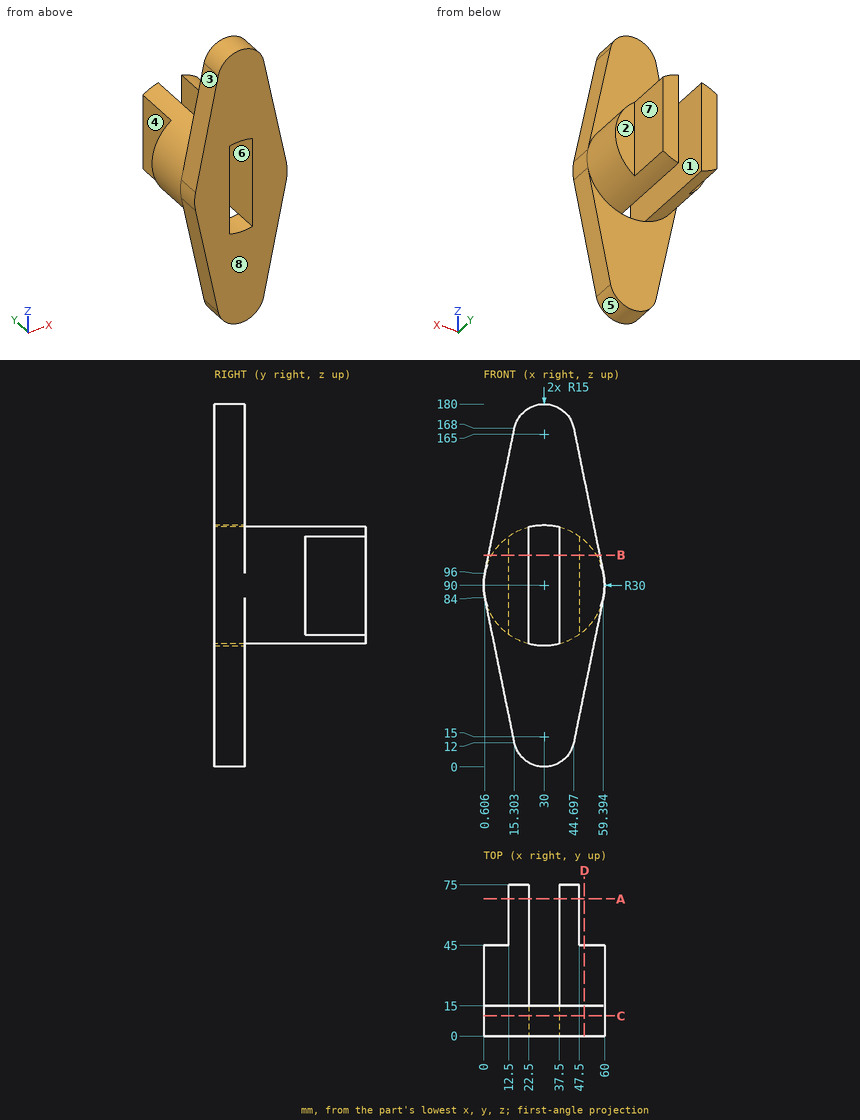
Here's the drawing with two shaded views (mm, measured from the low corner). I have some questions. A direction names the side the tool comes from. Round coordinates to 2 decimals unless told otherwise and drop trailing zeros. Order: outer loops, then holes, each group sorted by start corner. A loop starts at its lowest first (then second) coordinate and runs counter-clockwise, first axis right, second up. Notation, with made-up numbers: M 5.5,6.25 L 15.5,6.25 A18 cw 15.5,14.25 Z; hole C -39,61 d10. An arc over 180 degrees is marked long. Answer in a Markdown table with one row per item.
Item 1: If I drill on L1, parallel to X at y = 51, z = 114; L2, parallel to Y at x = 56.5, z = 86; L3, parallel to Y at x = 8, z = 121, over which ranges is the centre line in solid material (lowest first)? Write a range as from..to.
A:
| item | result |
|---|---|
| L1 | x = 12.5..22.5, 37.5..47.5 |
| L2 | y = 0..45 |
| L3 | y = 0..15 |
Item 2: Imagine slicing it at D-D, the plane x = 50. Write out the boundary of the cut face in (y, z), and give its area (3 significant figures).
A:
| item | result |
|---|---|
| outline | M 0,37.98 L 15,37.98 L 15,67.64 L 45,67.64 L 45,112.36 L 15,112.36 L 15,142.02 L 0,142.02 Z |
| area | 2,900 mm2 |
Item 3: Thinking about a two-plate mould opening in Z: for the marked faces 1, 2 and 3, which applies, +Z half, -Z half, draft (parallel to the pull), parting line (faces both ways), or undercut?
A:
| item | result |
|---|---|
| face 1 | undercut |
| face 2 | draft |
| face 3 | +Z half |
Item 4: Imagine slicing it at B-B, the plane z = 105. Write out the boundary of the cut face in (x, y), and give its area (3 significant figures).
A:
| item | result |
|---|---|
| outline | M 2.44,0 L 22.5,0 L 22.5,75 L 12.5,75 L 12.5,45 L 4.02,45 L 4.02,15 L 2.44,15 Z; M 37.5,0 L 57.56,0 L 57.56,15 L 55.98,15 L 55.98,45 L 47.5,45 L 47.5,75 L 37.5,75 Z |
| area | 2,310 mm2 |
Item 5: Imagine slicing it at C-C, the plane y = 10. Write out the boundary of the cut face in (x, z).
A:
| item | result |
|---|---|
| outline | M 0.61,84 L 15.3,12 A15 ccw 44.7,12 L 59.39,84 A30 ccw 59.39,96 L 44.7,168 A15 ccw 15.3,168 L 0.61,96 A30 ccw Z; hole M 22.5,60.95 A30 ccw 37.5,60.95 L 37.5,119.05 A30 ccw 22.5,119.05 Z |
Item 6: For the marked faces 4, 5, 6, 7 and 8, which set-ups out of +Z, -Z, +X, -X, +Y, -Y let a thin tool reach every point of the face, with its end or its side?
A:
| item | result |
|---|---|
| face 4 | +Z, -Z, -X, +Y |
| face 5 | -Z, +Y, -Y |
| face 6 | +Y, -Y |
| face 7 | +Z, -Z, +X, +Y |
| face 8 | +Z, -Z, +X, -X, -Y |
Item 7: I'm going to push flat-ended pins straight in: pin 1 (1 mm diameter, centred on x = 27, z = 139.5, fed in from -Y); pin 2 (15 mm diameter, centred on y = 54, z = 100.5, fed in from +X); pin 3 (4 mm diameter, centred on x = 52, z = 99.5, fed in from +Y); pin 4 (1.5 mm diameter, centred on x = 15, z = 126, fed in from +Y). Where does each tip first touch, or does it pass through?
A:
| item | result |
|---|---|
| pin 1 | stops at y = 0 |
| pin 2 | stops at x = 47.5 |
| pin 3 | stops at y = 45 |
| pin 4 | stops at y = 15 |
Item 8: Imagine slicing it at A-A, the plane y = 68. Write out the boundary of the cut face in (x, z).
A:
| item | result |
|---|---|
| outline | M 12.5,65.63 A30 ccw 22.5,60.95 L 22.5,119.05 A30 ccw 12.5,114.37 Z; M 37.5,60.95 A30 ccw 47.5,65.63 L 47.5,114.37 A30 ccw 37.5,119.05 Z |
